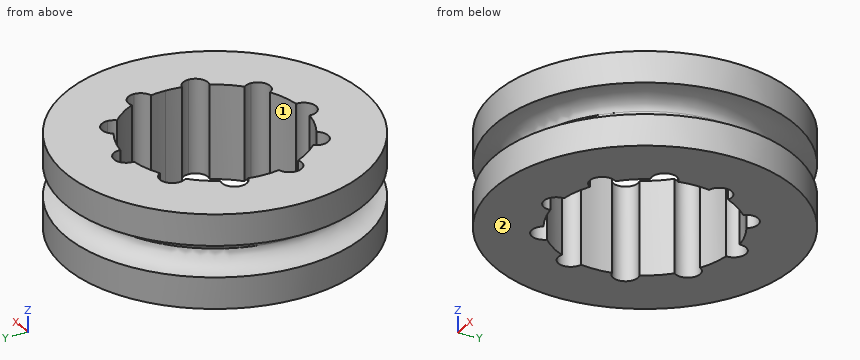
from build123d import *

# Parameters (mm, degrees)
F4_DEPTH = 9.907


with BuildPart() as f1:
    # F0 (on Front) → F1 (revolve)
    with BuildSketch(Plane.XZ):
        Polygon((0, 0), (0, 4.953), (-15.875, 4.953), (-15.875, 1.651), (-13.335, 1.651), (-13.335, 0), align=None)
        with BuildLine():
            Line((-13.335, 1.651), (-15.875, 1.651))
            add(Edge.make_bspline(
                [(-15.875, 1.651), (-14.605, 1.651), (-13.335, 0.8255), (-13.335, 0)],
                knots=[0, 0, 0, 0, 3.0294225522, 3.0294225522, 3.0294225522, 3.0294225522], degree=3))
            Line((-13.335, 0), (-13.335, 1.651))
        make_face()
    revolve(axis=Axis((0, 0, 11.7816049606), (0, 0, 1)))

    # F2: F1 across plane


with BuildPart() as f1_1:
    add(f1.part)
    add(f1.part.mirror(Plane.XY))

    # F3 (on face) → F4 (cut, through all)
    with BuildSketch(Plane.XY.offset(4.953)):
        with BuildLine():
            ThreePointArc((9.2166859434, -1.6310819203), (9.3240277448, -0.8186785842), (9.3599, 0))
            ThreePointArc((9.3599, 0), (9.3240277448, 0.8186785842), (9.2166859434, 1.6310819203))
            ThreePointArc((9.2166859434, 1.6310819203), (7.6654204157, 2.490646073), (8.4151814581, 4.0978590798))
            ThreePointArc((8.4151814581, 4.0978590798), (7.5723181657, 5.5016111829), (6.497729662, 6.7370050653))
            ThreePointArc((6.497729662, 6.7370050653), (4.737490355, 6.520596073), (4.3993636772, 8.2615571925))
            ThreePointArc((4.3993636772, 8.2615571925), (2.8923681657, 8.9017938869), (1.2968614994, 9.2696212577))
            ThreePointArc((1.2968614994, 9.2696212577), (0, 8.0599), (-1.2968614994, 9.2696212577))
            ThreePointArc((-1.2968614994, 9.2696212577), (-2.8923681657, 8.9017938869), (-4.3993636772, 8.2615571925))
            ThreePointArc((-4.3993636772, 8.2615571925), (-4.2520269006, 7.9308416953), (-4.2016111829, 7.5723181657))
            ThreePointArc((-4.2016111829, 7.5723181657), (-5.0571755986, 6.350648402), (-6.497729662, 6.7370050653))
            ThreePointArc((-6.497729662, 6.7370050653), (-7.5723181656, 5.5016111829), (-8.4151814581, 4.0978590798))
            ThreePointArc((-8.4151814581, 4.0978590798), (-7.824158476, 3.6194870839), (-7.6017938869, 2.8923681657))
            ThreePointArc((-7.6017938869, 2.8923681657), (-8.1015938099, 1.8678293246), (-9.2166859434, 1.6310819203))
            ThreePointArc((-9.2166859434, 1.6310819203), (-9.3599, 0), (-9.2166859434, -1.6310819203))
            ThreePointArc((-9.2166859434, -1.6310819203), (-8.1015938099, -1.8678293246), (-7.6017938869, -2.8923681657))
            ThreePointArc((-7.6017938869, -2.8923681657), (-7.824158476, -3.6194870839), (-8.4151814581, -4.0978590798))
            ThreePointArc((-8.4151814581, -4.0978590798), (-7.5723181656, -5.5016111829), (-6.497729662, -6.7370050653))
            ThreePointArc((-6.497729662, -6.7370050653), (-5.0571755986, -6.350648402), (-4.2016111829, -7.5723181657))
            ThreePointArc((-4.2016111829, -7.5723181657), (-4.2520269006, -7.9308416953), (-4.3993636772, -8.2615571925))
            ThreePointArc((-4.3993636772, -8.2615571925), (-2.8923681657, -8.9017938869), (-1.2968614994, -9.2696212577))
            ThreePointArc((-1.2968614994, -9.2696212577), (0, -8.0599), (1.2968614994, -9.2696212577))
            ThreePointArc((1.2968614994, -9.2696212577), (2.8923681657, -8.9017938869), (4.3993636772, -8.2615571925))
            ThreePointArc((4.3993636772, -8.2615571925), (4.737490355, -6.520596073), (6.497729662, -6.7370050653))
            ThreePointArc((6.497729662, -6.7370050653), (7.5723181657, -5.5016111829), (8.4151814581, -4.0978590798))
            ThreePointArc((8.4151814581, -4.0978590798), (7.6654204157, -2.490646073), (9.2166859434, -1.6310819203))
        make_face()
        with BuildLine():
            ThreePointArc((8.4151814581, 4.0978590798), (7.6654204157, 2.490646073), (9.2166859434, 1.6310819203))
            ThreePointArc((9.2166859434, 1.6310819203), (8.9017938869, 2.8923681657), (8.4151814581, 4.0978590798))
        make_face()
        with BuildLine():
            ThreePointArc((8.4151814581, 4.0978590798), (8.9017938869, 2.8923681657), (9.2166859434, 1.6310819203))
            ThreePointArc((9.2166859434, 1.6310819203), (9.9263327279, 2.0921680886), (10.2017938869, 2.8923681657))
            ThreePointArc((10.2017938869, 2.8923681657), (9.6289128051, 3.9700035765), (8.4151814581, 4.0978590798))
        make_face()
        with BuildLine():
            ThreePointArc((10.2017938869, -2.8923681657), (9.9263327279, -2.0921680886), (9.2166859434, -1.6310819203))
            ThreePointArc((9.2166859434, -1.6310819203), (8.9017938869, -2.8923681657), (8.4151814581, -4.0978590798))
            ThreePointArc((8.4151814581, -4.0978590798), (9.6289128051, -3.9700035765), (10.2017938869, -2.8923681657))
        make_face()
        with BuildLine():
            ThreePointArc((8.4151814581, -4.0978590798), (8.9017938869, -2.8923681657), (9.2166859434, -1.6310819203))
            ThreePointArc((9.2166859434, -1.6310819203), (7.6654204157, -2.490646073), (8.4151814581, -4.0978590798))
        make_face()
        with BuildLine():
            ThreePointArc((4.3993636772, 8.2615571925), (4.737490355, 6.520596073), (6.497729662, 6.7370050653))
            ThreePointArc((6.497729662, 6.7370050653), (5.5016111829, 7.5723181657), (4.3993636772, 8.2615571925))
        make_face()
        with BuildLine():
            ThreePointArc((4.3993636772, 8.2615571925), (5.5016111829, 7.5723181657), (6.497729662, 6.7370050653))
            ThreePointArc((6.497729662, 6.7370050653), (6.7232809466, 7.1278825813), (6.8016111829, 7.5723181657))
            ThreePointArc((6.8016111829, 7.5723181657), (5.8601347126, 8.821902448), (4.3993636772, 8.2615571925))
        make_face()
        with BuildLine():
            ThreePointArc((6.8016111829, -7.5723181657), (6.7232809466, -7.1278825813), (6.497729662, -6.7370050653))
            ThreePointArc((6.497729662, -6.7370050653), (5.5016111829, -7.5723181657), (4.3993636772, -8.2615571925))
            ThreePointArc((4.3993636772, -8.2615571925), (5.8601347126, -8.821902448), (6.8016111829, -7.5723181657))
        make_face()
        with BuildLine():
            ThreePointArc((4.3993636772, -8.2615571925), (5.5016111829, -7.5723181657), (6.497729662, -6.7370050653))
            ThreePointArc((6.497729662, -6.7370050653), (4.737490355, -6.520596073), (4.3993636772, -8.2615571925))
        make_face()
        with BuildLine():
            ThreePointArc((-1.2968614994, 9.2696212577), (0, 8.0599), (1.2968614994, 9.2696212577))
            ThreePointArc((1.2968614994, 9.2696212577), (0, 9.3599), (-1.2968614994, 9.2696212577))
        make_face()
        with BuildLine():
            ThreePointArc((-1.2968614994, 9.2696212577), (0, 9.3599), (1.2968614994, 9.2696212577))
            ThreePointArc((1.2968614994, 9.2696212577), (1.2992151379, 9.3147333599), (1.3, 9.3599))
            ThreePointArc((1.3, 9.3599), (-0.0451666401, 10.6591151379), (-1.2968614994, 9.2696212577))
        make_face()
        with BuildLine():
            ThreePointArc((1.3, -9.3599), (1.2992151379, -9.3147333599), (1.2968614994, -9.2696212577))
            ThreePointArc((1.2968614994, -9.2696212577), (0, -9.3599), (-1.2968614994, -9.2696212577))
            ThreePointArc((-1.2968614994, -9.2696212577), (-0.0451666401, -10.6591151379), (1.3, -9.3599))
        make_face()
        with BuildLine():
            ThreePointArc((-1.2968614994, -9.2696212577), (0, -9.3599), (1.2968614994, -9.2696212577))
            ThreePointArc((1.2968614994, -9.2696212577), (0, -8.0599), (-1.2968614994, -9.2696212577))
        make_face()
        with BuildLine():
            ThreePointArc((-4.2016111829, 7.5723181657), (-4.2520269006, 7.9308416953), (-4.3993636772, 8.2615571925))
            ThreePointArc((-4.3993636772, 8.2615571925), (-5.5016111829, 7.5723181657), (-6.497729662, 6.7370050653))
            ThreePointArc((-6.497729662, 6.7370050653), (-5.0571755986, 6.350648402), (-4.2016111829, 7.5723181657))
        make_face()
        with BuildLine():
            ThreePointArc((-6.497729662, 6.7370050653), (-5.5016111829, 7.5723181657), (-4.3993636772, 8.2615571925))
            ThreePointArc((-4.3993636772, 8.2615571925), (-6.2657320109, 8.6240402583), (-6.497729662, 6.7370050653))
        make_face()
        with BuildLine():
            ThreePointArc((-6.497729662, -6.7370050653), (-6.2657320109, -8.6240402583), (-4.3993636772, -8.2615571925))
            ThreePointArc((-4.3993636772, -8.2615571925), (-5.5016111829, -7.5723181657), (-6.497729662, -6.7370050653))
        make_face()
        with BuildLine():
            ThreePointArc((-6.497729662, -6.7370050653), (-5.5016111829, -7.5723181657), (-4.3993636772, -8.2615571925))
            ThreePointArc((-4.3993636772, -8.2615571925), (-4.2520269006, -7.9308416953), (-4.2016111829, -7.5723181657))
            ThreePointArc((-4.2016111829, -7.5723181657), (-5.0571755986, -6.350648402), (-6.497729662, -6.7370050653))
        make_face()
        with BuildLine():
            ThreePointArc((-7.6017938869, 2.8923681657), (-7.824158476, 3.6194870839), (-8.4151814581, 4.0978590798))
            ThreePointArc((-8.4151814581, 4.0978590798), (-8.9017938869, 2.8923681657), (-9.2166859434, 1.6310819203))
            ThreePointArc((-9.2166859434, 1.6310819203), (-8.1015938099, 1.8678293246), (-7.6017938869, 2.8923681657))
        make_face()
        with BuildLine():
            ThreePointArc((-9.2166859434, 1.6310819203), (-8.9017938869, 2.8923681657), (-8.4151814581, 4.0978590798))
            ThreePointArc((-8.4151814581, 4.0978590798), (-10.1381673581, 3.2940902583), (-9.2166859434, 1.6310819203))
        make_face()
        with BuildLine():
            ThreePointArc((-9.2166859434, -1.6310819203), (-10.1381673581, -3.2940902583), (-8.4151814581, -4.0978590798))
            ThreePointArc((-8.4151814581, -4.0978590798), (-8.9017938869, -2.8923681657), (-9.2166859434, -1.6310819203))
        make_face()
        with BuildLine():
            ThreePointArc((-9.2166859434, -1.6310819203), (-8.9017938869, -2.8923681657), (-8.4151814581, -4.0978590798))
            ThreePointArc((-8.4151814581, -4.0978590798), (-7.824158476, -3.6194870839), (-7.6017938869, -2.8923681657))
            ThreePointArc((-7.6017938869, -2.8923681657), (-8.1015938099, -1.8678293246), (-9.2166859434, -1.6310819203))
        make_face()
    extrude(amount=-F4_DEPTH, mode=Mode.SUBTRACT)


solid = f1_1.part
For this review, take the finished solid that the model builds, in its own axes (mm). Face numbers are marked on the shaded views. A direction names the side the tool comes from. Round coordinates to 2 decimals unless told otherwise and drop trailing zeros. Write item = value, one per line. Start each with the question number.
1) Insertion check: pin 1 (1 mm diameter, centred on y = 9.5, z = 0, fed in from -X). The pin has a flat end and moves straight along its axis. Give the tip position at first contact, or say it passes through.
2) To check wall thickness, follow line 1 (Y direction, x = -9.5, z = 2.25); line 2 (Y direction, x = 7.5, z = -3.5); line 3 (Z direction, x = -8, y = -13.5). State the ranges of each line that lie inside material, in increasing order. Write a range as from..to.
3) Tool access review of the marked faces 1 and 2: name each direction out of +Z, -Z, +X, -X, +Y, -Y from which nothing blocks a thin tool from reaching the whole face with its end or side.
Verdict:
q1.pin_1 = -9.84
q2.line_1 = -12.72..-4.05, -1.74..1.74, 4.05..12.72
q2.line_2 = -13.99..-5.6, 5.6..13.99
q2.line_3 = -4.95..-1.65, 1.65..4.95
q3.face_1 = +Z, -Z
q3.face_2 = -Z, +X, -X, +Y, -Y
